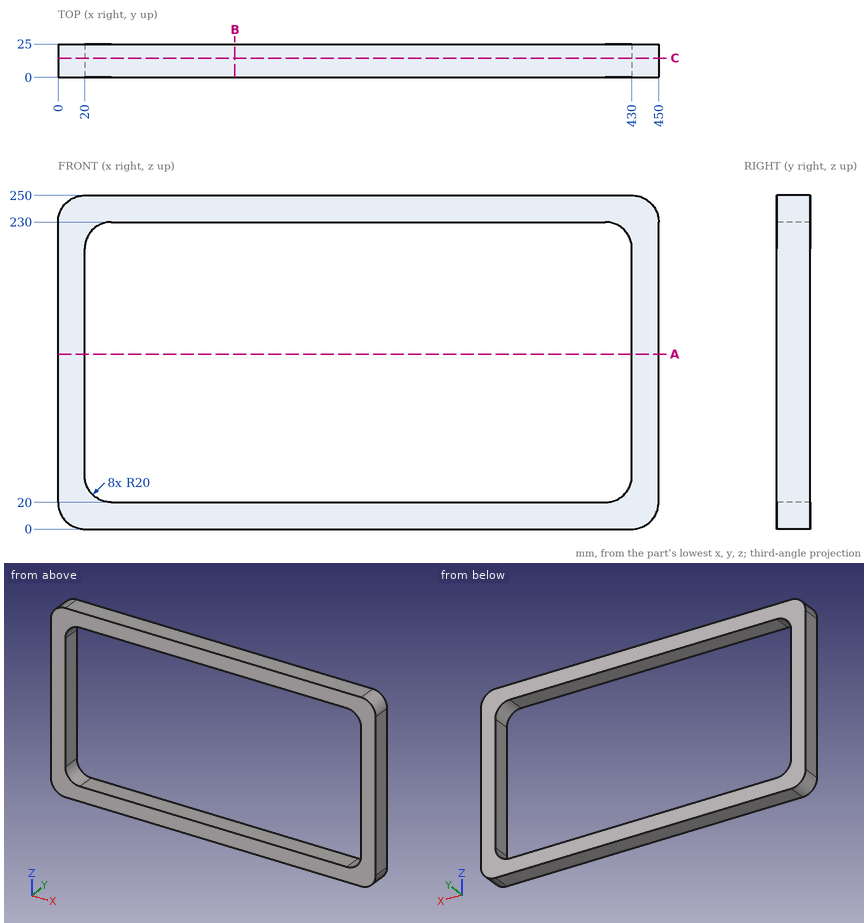
Answer from the drawing. Dimensions are ordinates in mm from the lowest x, y and z of the part. Round coordinates to 2 decimals unless told otherwise and drop trailing zeros. Loops run counter-clockwise (first coordinate to the right, second up) from the corner with the lowest first, then second, coordinate; pieces in that order, holes last.
1) Consider line 1 (X direction, y = 12, z = 190); line 2 (Z direction, x = 144, y = 10); line 3 (X direction, y = 22, z = 24.5). Determine where each line is inside the solid, lowest interval first.
Outcome:
line 1: x = 0 to 20, 430 to 450
line 2: z = 0 to 20, 230 to 250
line 3: x = 0 to 27.36, 422.64 to 450
2) A cutting plane is placed at B-B on x = 132.5. Determine the outline of the cut face in (y, z).
Outcome:
outline: (0, 0) - (25, 0) - (25, 20) - (0, 20) - close; (0, 230) - (25, 230) - (25, 250) - (0, 250) - close
3) A cutting plane is placed at A-A on z = 131. Determine the outline of the cut face in (x, y).
Outcome:
outline: (0, 0) - (20, 0) - (20, 25) - (0, 25) - close; (430, 0) - (450, 0) - (450, 25) - (430, 25) - close
4) A cutting plane is placed at C-C on y = 14.5. Determine the outline of the cut face in (x, z).
Outcome:
outline: (0, 20) arc R20 ccw to (20, 0) - (430, 0) arc R20 ccw to (450, 20) - (450, 230) arc R20 ccw to (430, 250) - (20, 250) arc R20 ccw to (0, 230) - close; hole (20, 40) arc R20 ccw to (40, 20) - (410, 20) arc R20 ccw to (430, 40) - (430, 210) arc R20 ccw to (410, 230) - (40, 230) arc R20 ccw to (20, 210) - close
